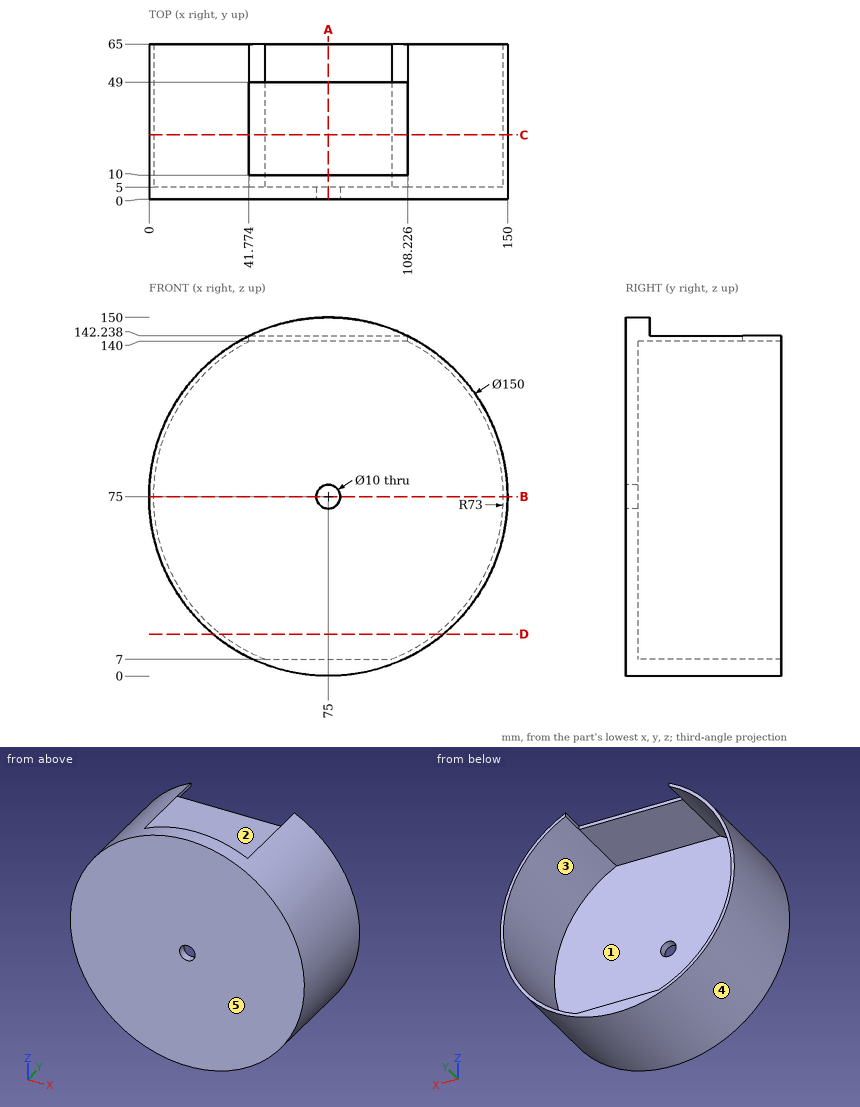
For this review, use the dimensioned drawing (mm, ordinates from the lowest corner) and the shaded views. A direction names the side the tool comes from. Coordinates: 2 decimals unless noted, no trailing zeros. Loops run counter-clockwise (first coordinate to the right, second up) from the corner with the lowest first, then second, coordinate; pieces in that order, holes last.
1. Mouldability with a two-part tool opening along X and no side actions: class the marked faces 3, 4 and 5 as +X half, -X half, draft (parallel to the pull), parting line (faces both ways), or undercut.
2. For line 1 (X direction, y = 2.35, z = 75); line 2 (Y direction, x = 34.5, z = 21.5); line 3 (X direction, y = 6, z = 94.5), list the stretches that pass through material, from the lowest coordinate up.
3. Add section C-C, the plane y = 27. Give the boundary of the cut face in (x, z), then the cut area to 3 significant figures.
4. Add section B-B, the plane z = 75. Give the boundary of the cut face in (x, y).
5. Add section D-D, the plane z = 17.5. Give the boundary of the cut face in (x, y) (1 decimal), then the cut area to 3 significant figures.
6. For the marked faces 1 and 2, list the 3-axis set-ups (+Z, -Z, +X, -X, +Y, -Y) from which the entire face can be reached by the end or side of a thin tool; tool diameter is ignored.
7. Add section A-A, the plane x = 75. Give the boundary of the cut face in (y, z), then the cut area to 3 significant figures.
8. Insertion check: P1, Ø0.7, axis at x = 66, z = 140.5, coming from the +Y side; P2, Ø10, axis at y = 9, z = 43.5, coming from the +X side; P3, Ø6, axis at x = 63, y = 24, coming from the -Z side. Each pin has a flat end and moves straight along its axis. Give the tip position at first contact, or say it passes through.
Result:
1. face 3: undercut
1. face 4: parting line
1. face 5: draft
2. line 1: x = 0 to 70, 80 to 150
2. line 2: y = 0 to 5
2. line 3: x = 2.58 to 4.65, 145.35 to 147.42
3. outline: (41.77, 142.24) arc R75 ccw (long way) to (108.23, 142.24) - close; hole (41.77, 140) arc R73 ccw to (48.45, 7) - (101.55, 7) arc R73 ccw to (108.23, 140) - close
3. area: 1,120 mm2
4. outline: (0, 0) - (70, 0) - (70, 5) - (2, 5) - (2, 65) - (0, 65) - close; (80, 0) - (150, 0) - (150, 65) - (148, 65) - (148, 5) - (80, 5) - close
5. outline: (26.8, 0) - (123.2, 0) - (123.2, 65) - (120, 65) - (120, 5) - (30, 5) - (30, 65) - (26.8, 65) - close
5. area: 863 mm2
6. face 1: +Y
6. face 2: +Z, +X, -X, +Y
7. outline: (0, 0) - (65, 0) - (65, 7) - (5, 7) - (5, 70) - (0, 70) - close; (0, 80) - (5, 80) - (5, 140) - (49, 140) - (49, 142.24) - (10, 142.24) - (10, 150) - (0, 150) - close
7. area: 1,260 mm2
8. P1: stops at y = 49
8. P2: stops at x = 145.16
8. P3: stops at z = 0.54
